Here's how the part is built. I have some questions about the finished solid (model axes, mm). A direction names the side the tool comes from. Coordinates: 2 decimals unless noted, no trailing zeros. Loops run counter-clockwise (first coordinate to the right, second up) from the corner with the lowest first, then second, coordinate; pieces in that order, holes last. Notation, with made-up numbers: (45, 9) - (94, 9) arc R6 cw to (94, 20) - close; hole circle Ø7 at (13.5, -14.5). An arc over 180 degrees is marked (long way). Use a Markdown table: item, result.
```python
from build123d import *

# Parameters (mm, degrees)
SKETCH1_W           = 30
SKETCH1_H           = 36
BOSS_EXTRUDE1_DEPTH = 9
CUT_EXTRUDE1_DEPTH  = 37
SKETCH3_W           = 22
SKETCH3_H           = 7
CUT_EXTRUDE2_DEPTH  = 16.5
SKETCH4_W           = 14
SKETCH4_H           = 7
CUT_EXTRUDE3_DEPTH  = 20.5
BOSS_EXTRUDE4_DEPTH = 36
SKETCH6_R           = 6
CUT_EXTRUDE4_DEPTH  = 37
CUT_EXTRUDE8_DEPTH  = 4
SKETCH8_R           = 2.5
CUT_EXTRUDE9_DEPTH  = 3
SKETCH9_R           = 0.6
CUT_EXTRUDE10_DEPTH = 31


with BuildPart() as part:
    # Sketch1 → Boss-Extrude1 (new body)
    with BuildSketch(Plane(origin=(0, 0, 0), x_dir=(1, 0, 0), z_dir=(0, 1, 0))):
        Rectangle(SKETCH1_W, SKETCH1_H)
    extrude(amount=BOSS_EXTRUDE1_DEPTH)

    # Sketch2 → Cut-Extrude1 (cut, through all)
    with BuildSketch(Plane.XY.offset(18)):
        Polygon((-12, 0), (-13, 2.1), (-8.8, 2.1), (-9.8, 0), align=None)
        Polygon((12, 0), (13, 2.1), (8.8, 2.1), (9.8, 0), align=None)
    extrude(amount=-CUT_EXTRUDE1_DEPTH, mode=Mode.SUBTRACT)

    # Sketch3 → Cut-Extrude2 (cut)
    with BuildSketch(Plane.XY.offset(18)):
        with Locations((4, 3.5)):
            Rectangle(SKETCH3_W, SKETCH3_H)
    extrude(amount=-CUT_EXTRUDE2_DEPTH, mode=Mode.SUBTRACT)

    # Sketch4 → Cut-Extrude3 (cut, through all)
    with BuildSketch(Plane.XY.offset(1.5)):
        with Locations((0, 3.5)):
            Rectangle(SKETCH4_W, SKETCH4_H)
    extrude(amount=-CUT_EXTRUDE3_DEPTH, mode=Mode.SUBTRACT)

    # Sketch5 → Boss-Extrude4 (add)
    with BuildSketch(Plane.XY.offset(18)):
        with BuildLine():
            Line((-4.898979486, 9), (4.898979486, 9))
            ThreePointArc((4.898979486, 9), (7.986516373, 14.860274987), (5.598833698, 21.038841035))
            Line((5.598833698, 21.038841035), (5.598833698, 26.038841035))
            Line((5.598833698, 26.038841035), (-5.598833698, 26.038841035))
            Line((-5.598833698, 26.038841035), (-5.598833698, 21.038841035))
            ThreePointArc((-5.598833698, 21.038841035), (-7.986516373, 14.860274987), (-4.898979486, 9))
        make_face()
    extrude(amount=-BOSS_EXTRUDE4_DEPTH)

    # Sketch6 → Cut-Extrude4 (cut, through all)
    with BuildSketch(Plane(origin=(0, 0, -18), x_dir=(-1, 0, 0), z_dir=(0, 0, -1))):
        with Locations((0, 15.32455532)):
            Circle(SKETCH6_R)
    extrude(amount=-CUT_EXTRUDE4_DEPTH, mode=Mode.SUBTRACT)

    # Sketch7 → Cut-Extrude8 (cut)
    with BuildSketch(Plane(origin=(0, 26.038841035, 0), x_dir=(1, 0, 0), z_dir=(0, 1, 0))):
        Polygon((2.3, -3.983716857), (4.6, 0), (2.3, 3.983716857), (-2.3, 3.983716857), (-4.6, 0), (-2.3, -3.983716857), align=None)
    extrude(amount=-CUT_EXTRUDE8_DEPTH, mode=Mode.SUBTRACT)

    # Sketch8 → Cut-Extrude9 (cut)
    with BuildSketch(Plane(origin=(0, 22.038841035, 0), x_dir=(1, 0, 0), z_dir=(0, 1, 0))):
        Circle(SKETCH8_R)
    extrude(amount=-CUT_EXTRUDE9_DEPTH, mode=Mode.SUBTRACT)

    # Sketch9 → Cut-Extrude10 (cut, through all)
    with BuildSketch(Plane.ZY.offset(15)):
        with Locations((-18, 3)):
            Circle(SKETCH9_R)
    extrude(amount=-CUT_EXTRUDE10_DEPTH, mode=Mode.SUBTRACT)


solid = part.part
```
Q1. If we mould it in two halves opening along X, with no side actions, what happens to faces 1 (the face through (-5.599, 24, 0)), 2 (the face through (-3.4, 10.1, 18)), 3 (the face through (-9.293, 1.065, 0.252))? For each: pulls with the +X half, pulls with the -X half, needs draft (parallel to the pull), parting line crosses it, or undercut.
Check values:
| item | result |
|---|---|
| face 1 | pulls with the -X half |
| face 2 | needs draft |
| face 3 | undercut |
Q2. I want a section at D-D, the plane x = -11.5. Write out the boundary of the cut face in (y, z), then the cut area to 3 significant figures.
Check values:
| item | result |
|---|---|
| outline | (2.1, -18) - (2.4, -18) arc R0.6 cw to (3.6, -18) - (9, -18) - (9, 18) - (2.1, 18) - close |
| area | 248 mm^2 |
Q3. I want a section at A-A, the plane y = 3. Write out the boundary of the cut face in (x, z), then the cut area to 3 significant figures.
Check values:
| item | result |
|---|---|
| outline | (-15, -17.4) - (-7, -17.4) - (-7, 18) - (-15, 18) - close; (7, -17.4) - (15, -17.4) - (15, 1.5) - (7, 1.5) - close |
| area | 434 mm^2 |
Q4. Please list where these lines run through material, in increasing order: L1, parallel to X at y = 15, z = 5; L2, parallel to Z at x = 0, y = 21.8; L3, parallel to X at y = 21.05, z = 0. Write a range as from..to.
Check values:
| item | result |
|---|---|
| L1 | -7.99..-5.99, 5.99..7.99 |
| L2 | -18..-2.5, 2.5..18 |
| L3 | -5.6..-2.5, 2.5..5.6 |
Q5. I want a section at C-C, the plane z = 9.5. Write out the boundary of the cut face in (x, y), then the cut area to 3 significant figures.
Check values:
| item | result |
|---|---|
| outline | (-15, 0) - (-12, 0) - (-13, 2.1) - (-8.8, 2.1) - (-9.8, 0) - (-7, 0) - (-7, 7) - (15, 7) - (15, 9) - (4.9, 9) arc R8 ccw to (5.6, 21.04) - (5.6, 26.04) - (-5.6, 26.04) - (-5.6, 21.04) arc R8 ccw to (-4.9, 9) - (-15, 9) - close; hole circle Ø12 at (0, 15.32) |
| area | 224 mm^2 |
Q6. Which directions (+Z, -Z, +X, -X, +Y, -Y) give clear straight access to the entire face, cutting with the end or side of a thin tool? Please do faces 4 (the face through (11, 4, 1.5)), 5 (the face through (10, 9, 0)), 6 (the face through (2, 22.039, -2)), 7 (the face through (11, 2.1, -8)).
Check values:
| item | result |
|---|---|
| face 4 | +Z, +X, -Y |
| face 5 | +Z, -Z, +X |
| face 6 | +Y |
| face 7 | +Z, -Z |
Q7. I want a section at B-B, the plane x = 0. Write out the boundary of the cut face in (y, z).
Check values:
| item | result |
|---|---|
| outline | (7, -18) - (9.32, -18) - (9.32, 18) - (7, 18) - close; (21.32, -18) - (26.04, -18) - (26.04, -3.98) - (22.04, -3.98) - (22.04, -2.5) - (21.32, -2.5) - close; (21.32, 2.5) - (22.04, 2.5) - (22.04, 3.98) - (26.04, 3.98) - (26.04, 18) - (21.32, 18) - close |
Q8. Will these pins go through, and if not, where does the flat tip stop? P1, Ø4, axis at x = -1.5, z = -0.5, coming from the -Y side; P2, Ø6, axis at x = 0, z = 0, coming from the +Y side; P3, Ø5.5, axis at x = 11.5, y = 3.5, coming from the +Z side.
Check values:
| item | result |
|---|---|
| P1 | y = 7 |
| P2 | y = 22.04 |
| P3 | z = 1.5 |
